For this review, take the finished solid that the model builds, in its own axes (mm). Face numbers are marked on the shaded views. A direction names the side the tool comes from. Coordinates: 2 decimals unless noted, no trailing zeros. Order: outer loops, then holes, each group sorted by start corner. A loop starts at its lowest first (then second) coordinate and runs counter-clockwise, first axis right, second up. Notation, with made-up numbers: (83.5, -33.5) -> (90.5, -33.5) arc R29 ccw to (90.5, -0.5) -> close; hole circle Ø4 at (42, -31.75). An arc over 180 degrees is marked (long way). Return JSON: item names as keys, results as strings. Group by question number.
Item 1: Take a section at A-A (y = 26). Write out the cut boundary in (x, z), then the cut area to 3 significant figures.
Item 2: Take a section at B-B (x = -15). Write out the cut boundary in (y, z).
Item 3: For line 1 along Y through (x, z) = (5, 0); line 2 along X through (y, z) = (11.5, 13); line 3 along X through (y, z) = (4.2, 0), list the stretches that pass through material, from the lowest coordinate up.
Item 4: Take a section at C-C (z = 0). Count the separate pieces of the cut face and the enclosed holes in it, then the cut area to 3 significant figures.
Item 5: Draft analysis for pull direction Z (two halves, no side actions). For the marked faces 1 and 2, state which applies: +Z half, -Z half, draft (parallel to the pull), parting line (faces both ways), or undercut.
Item 6: Machinability: for the marked faces 3 and 4, which of the approach directions +Z, -Z, +X, -X, +Y, -Y give a long, thin tool a straight path to every point of the face, cutting with its end or side? Answer none if there is none.
Item 7: Insertion check: pin 1 (7.5 mm diameter, centred on y = 22.5, z = 3.5, fed in from -X); pin 2 (2 mm diameter, centred on x = -6.5, y = 26, fed in from +Z); pin 3 (8 mm diameter, centred on x = -7, z = 20, fed in from +Y); pin 4 (1.5 mm diameter, centred on x = -15, z = 0, fed in from -Y). Each pin has a flat end and moves straight along its axis. Give the tip position at first contact, or say it passes through.
Item 8: Take a section at D-D (y = 9). Write out the cut boundary in (x, z).
Autodesk Inventor part; units mm, degrees
ref_plane "Work Plane1" through (6.5, 0, 0) normal (1, 0, 0) x (0, 1, 0)
ref_plane "Work Plane2" through (0, 30, 0) normal (0, 1, 0) x (-1, 0, 0)
ref_plane "XY Plane" through (0, 0, 0) normal (0, 0, 1) x (1, 0, 0)
sketch "Sketch1" plane through (0, 0, 0) normal (1, 0, 0) x (0, 1, 0)
  arc A0 (0, -30) -> (30, 0) centre (0, 0) ccw
  line L0 (30, 0) -> (0, 0)
  line L1 (0, 0) -> (0, -30)
  dimension "d0" = 30
revolve "Revolution1" add sketch "Sketch1" angle 360 about axis through (0, 30, 0) along (0, -1, 0)
ref_plane "Work Plane1" through (6.5, 0, 0) normal (1, 0, 0) x (0, 1, 0)
sketch "Sketch3" plane through (6.5, 0, 0) normal (1, 0, 0) x (0, 1, 0)
  circle A0 centre (30, 0) radius 25
  line L0 (0, 30) -> (0, -30)
  point P0 (0, 0)
  dimension "d7" = 50
  dimension "d8" = 30
extrude "Extrusion2" cut sketch "Sketch3" along normal through all
mirror "Mirror1" about plane through (0, 0, 0) normal (1, 0, 0) of "Extrusion2"
sketch "Sketch4" plane through (0, 0, 0) normal (1, 0, 0) x (0, 1, 0)
  arc A0 (0, -30) -> (0, 30) centre (0, 0) ccw
  circle A1 centre (30, 0) radius 25
  dimension "d11" = 50
extrude "Extrusion3" cut sketch "Sketch4" along normal mid plane 3
sketch "Sketch5" plane through (6.5, 0, 0) normal (1, 0, 0) x (0, 0, -1)
  circle A0 centre (0, 15) radius 2.5
  line L0 (-30, 0) -> (30, 0)
  point P0 (0, 0)
  dimension "d14" = 5
  dimension "d15" = 15
extrude "Extrusion4" cut sketch "Sketch5" against normal through all
ref_plane "Work Plane2" through (0, 30, 0) normal (0, 1, 0) x (-1, 0, 0)
sketch "Sketch7" plane through (0, 30, 0) normal (0, 1, 0) x (-1, 0, 0)
  line L0 (15, 0) -> (-15, 0) construction
  point P0 (0, 0)
  point P1 (0, 0)
  dimension "d21" = 30
hole "Hole1" at (-15, 30, 0) at (15, 30, 0) direction (0, -1, 0) diameter 2.5 end through all counterbore diameter 5 counterbore depth 27.5
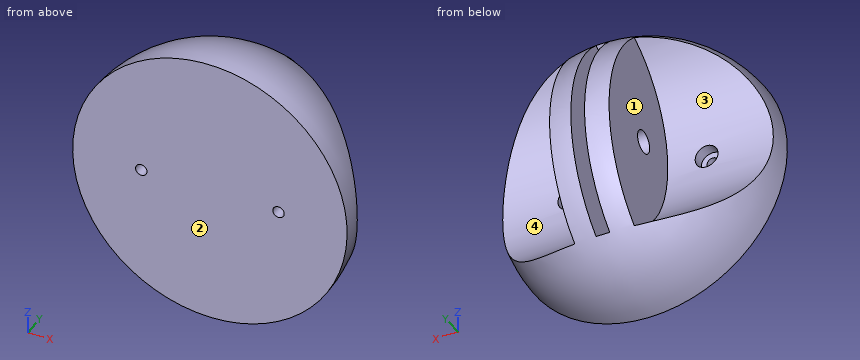
Findings below:
{
 "1": {"outline": "(-6.5, -13.48) arc R14.97 ccw to (-1.5, -14.89) -> (-1.5, 14.89) arc R14.97 ccw to (-6.5, 13.48) -> close; (1.5, -14.89) arc R14.97 ccw to (6.5, -13.48) -> (6.5, 13.48) arc R14.97 ccw to (1.5, 14.89) -> close", "area": "287 mm2"},
 "2": {"outline": "(0, -25.98) arc R25.98 ccw to (15.83, -20.6) arc R25 cw to (5.13, -2.5) -> (2.5, -2.5) -> (2.5, -1.25) -> (0, -1.25) -> close; (0, 1.25) -> (2.5, 1.25) -> (2.5, 2.5) -> (5.13, 2.5) arc R25 cw to (15.83, 20.6) arc R25.98 ccw to (0, 25.98) -> close"},
 "3": {"line 1": "y = 0 to 12.5, 17.5 to 29.58", "line 2": "x = -6.5 to -1.5, 1.5 to 6.5", "line 3": "x = -29.7 to -17.5, -12.5 to 12.5, 17.5 to 29.7"},
 "4": {"separate pieces": "5", "enclosed holes": "0", "area": "458 mm2"},
 "5": {"face 1": "undercut", "face 2": "draft"},
 "6": {"face 3": "-X, +Y", "face 4": "+X, +Y"},
 "7": {"pin 1": "stops at x = -6.5", "pin 2": "stops at z = 15.31", "pin 3": "stops at y = 24.59", "pin 4": "passes through"},
 "8": {"outline": "(-25.2, -13.56) arc R28.62 ccw to (25.2, -13.56) -> (6.5, -13.56) -> (6.5, 13.56) -> (25.2, 13.56) arc R28.62 ccw to (-25.2, 13.56) -> (-6.5, 13.56) -> (-6.5, -13.56) -> close; hole (-1.5, -13.56) -> (1.5, -13.56) -> (1.5, 13.56) -> (-1.5, 13.56) -> close"}
}
